Design review of the part built by this model. Coordinates are the model's own, in mm. Give positions to 0.01 mm unless a question says otherwise; leave off trailing zeros. Order: outer loops, then holes, each group sorted by start corner. A loop starts at its lowest first (then second) coordinate and runs counter-clockwise, first axis right, second up. Notation, with made-up numbers: (-10.5, 76.25) - (38.5, 76.25) arc R17 cw to (38.5, 90.25) - close; hole circle Ø6 at (-2.5, 63). An arc over 180 degrees is marked (long way). Write each question's results on one line, items separated by ' | '. Start each with the question number.
```python
from build123d import *

# Parameters (mm, degrees)
SKETCH2_W           = 106
SKETCH2_H           = 106
SKETCH2_R           = 4
SKETCH2_R_2         = 6
BOSS_EXTRUDE1_DEPTH = 25
SKETCH3_W           = 106
SKETCH3_H           = 106
SKETCH3_W_2         = 100
SKETCH3_H_2         = 100
BOSS_EXTRUDE2_DEPTH = 20
SKETCH5_W           = 3
SKETCH5_H           = 23
BOSS_EXTRUDE3_DEPTH = 20
SKETCH7_W           = 20
SKETCH7_H           = 3
BOSS_EXTRUDE4_DEPTH = 20
SKETCH9_R           = 9.905763918
CUT_EXTRUDE1_DEPTH  = 10
SKETCH10_W          = 10
SKETCH10_H          = 4
BOSS_EXTRUDE5_DEPTH = 10
SKETCH11_W          = 10
SKETCH11_H          = 4
BOSS_EXTRUDE6_DEPTH = 10
FILLET2_RADIUS      = 5
FILLET2_LENGTH      = 4
FILLET3_R           = 5
FILLET4_R           = 5
FILLET5_R           = 5
SKETCH13_R          = 1.6
CUT_EXTRUDE2_DEPTH  = 163.397660082
SKETCH14_W          = 35.96051594
SKETCH14_H          = 7.693498276
CUT_EXTRUDE3_DEPTH  = 30


with BuildPart() as part:
    # Sketch2 → Boss-Extrude1 (new body)
    with BuildSketch(Plane(origin=(0, 0, 0), x_dir=(1, 0, 0), z_dir=(0, 1, 0))):
        with Locations((53, 53)):
            Rectangle(SKETCH2_W, SKETCH2_H)
        with Locations(Location((18, 15, 0), (0, 0, 270))):
            Circle(SKETCH2_R, mode=Mode.SUBTRACT)
        with Locations(Location((92, 13.5, 0), (0, 0, 270))):
            Circle(SKETCH2_R_2, mode=Mode.SUBTRACT)
    extrude(amount=BOSS_EXTRUDE1_DEPTH)

    # Sketch3 → Boss-Extrude2 (add)
    with BuildSketch(Plane(origin=(0, 25, 0), x_dir=(1, 0, 0), z_dir=(0, 1, 0))):
        with Locations((53, 53)):
            Rectangle(SKETCH3_W, SKETCH3_H)
        with Locations((53, 53)):
            Rectangle(SKETCH3_W_2, SKETCH3_H_2, mode=Mode.SUBTRACT)
    extrude(amount=BOSS_EXTRUDE2_DEPTH)

    # Sketch5 → Boss-Extrude3 (add)
    with BuildSketch(Plane(origin=(0, 25, 0), x_dir=(1, 0, 0), z_dir=(0, 1, 0))):
        Polygon((3, 28), (3, 25), (36, 25), (36, 23), (39, 23), (39, 43), (36, 43), (36, 28), align=None)
        Polygon((83, 52.5), (83, 26.5), (76, 26.5), (76, 3), (73, 3), (73, 29.5), (80, 29.5), (80, 49.5), (73, 49.5), (73, 52.5), align=None)
        Polygon((3, 63), (3, 60), (29, 60), (29, 80), (26, 80), (26, 63), align=None)
        with Locations((57.5, 14.5)):
            Rectangle(SKETCH5_W, SKETCH5_H)
    extrude(amount=BOSS_EXTRUDE3_DEPTH)

    # Sketch7 → Boss-Extrude4 (add)
    with BuildSketch(Plane(origin=(0, 25, 0), x_dir=(1, 0, 0), z_dir=(0, 1, 0))):
        Polygon((50, 70.496538655), (53, 70.496538655), (53, 73.496538655), (53, 87.496538655), (50, 87.496538655), align=None)
        with Locations((63, 71.996538655)):
            Rectangle(SKETCH7_W, SKETCH7_H)
        Polygon((73, 70.496538655), (73, 52.5), (76, 52.5), (76, 86.5), (73, 86.5), (73, 73.496538655), align=None)
    extrude(amount=BOSS_EXTRUDE4_DEPTH)

    # Sketch9 → Cut-Extrude1 (cut)
    with BuildSketch(Plane(origin=(0, 25, 0), x_dir=(1, 0, 0), z_dir=(0, 1, 0))):
        with Locations(Location((92, 13.5, 0), (0, 0, 270))):
            Circle(SKETCH9_R)
    extrude(amount=-CUT_EXTRUDE1_DEPTH, mode=Mode.SUBTRACT)

    # Sketch10 → Boss-Extrude5 (add)
    with BuildSketch(Plane.XY):
        with Locations((53, 2)):
            Rectangle(SKETCH10_W, SKETCH10_H)
    extrude(amount=BOSS_EXTRUDE5_DEPTH)

    # Sketch11 → Boss-Extrude6 (add)
    with BuildSketch(Plane(origin=(0, 0, -106), x_dir=(-1, 0, 0), z_dir=(0, 0, -1))):
        with Locations((-53, 2)):
            Rectangle(SKETCH11_W, SKETCH11_H)
    extrude(amount=BOSS_EXTRUDE6_DEPTH)

    # Fillet2: full round fillet: the end face becomes a half cylinder, R = half its width
    fillet2_face = Plane((53, 2, -116), x_dir=(0, -1, 0), z_dir=(0, 0, -1))  # on the end face: x along it, z out of the body
    fillet2_slab = fillet2_face.offset(-FILLET2_RADIUS / 2) * Box(FILLET2_LENGTH, 2 * FILLET2_RADIUS, FILLET2_RADIUS, mode=Mode.PRIVATE)  # the body's end, R deep
    fillet2_round = Plane((53, 2, -111), x_dir=(0, 0, -1), z_dir=(0, -1, 0)) * Cylinder(FILLET2_RADIUS, FILLET2_LENGTH, mode=Mode.PRIVATE)  # its axis R under the face
    add(fillet2_slab - fillet2_round, mode=Mode.SUBTRACT)

    # Fillet3
    fillet3_edges = [part.edges().sort_by_distance(p)[0] for p in [
        (48, 2, -106),
        (58, 2, -106),
    ]]
    fillet(fillet3_edges, radius=FILLET3_R - 0.0001)  # a hair under: the kernel refuses the full size

    # Fillet4
    fillet4_edges = [part.edges().sort_by_distance(p)[0] for p in [
        (48, 2, 0),
        (58, 2, 0),
    ]]
    fillet(fillet4_edges, radius=FILLET4_R)

    # Fillet5
    fillet5_edges = [part.edges().sort_by_distance(p)[0] for p in [
        (48, 2, 10),
        (58, 2, 10),
    ]]
    fillet(fillet5_edges, radius=FILLET5_R - 0.0001)  # a hair under: the kernel refuses the full size

    # Sketch13 → Cut-Extrude2 (cut, through all)
    with BuildSketch(Plane(origin=(0, 4, 0), x_dir=(1, 0, 0), z_dir=(0, 1, 0))):
        with Locations(Location((53, -5, 0), (0, 0, 180))):
            Circle(SKETCH13_R)
        with Locations(Location((53, 111, 0), (0, 0, 180))):
            Circle(SKETCH13_R)
    extrude(amount=-CUT_EXTRUDE2_DEPTH, mode=Mode.SUBTRACT)

    # Sketch14 → Cut-Extrude3 (cut)
    with BuildSketch(Plane.XY):
        with Locations((88.01974203, 3.846749138)):
            Rectangle(SKETCH14_W, SKETCH14_H)
    extrude(amount=-CUT_EXTRUDE3_DEPTH, mode=Mode.SUBTRACT)


solid = part.part
```
Q1. Draft analysis for pull direction Z (two halves, no side actions). For faces 1 (the flat face through (3, 35, -14)), 2 (the flat face through (53, 4, 3)), 3 (the cylindrical face through (46, 2, 1)), state which applies: pulls with the +Z half, pulls with the -Z half, needs draft (parallel to the pull), parting line crosses it, or undercut.
Q2. Add section C-C (z = -13.5). Give the number of separate pieces and of enclosed holes in the cut face, plus the area to 3 significant figures.
Q3. Insertion check: pin 1 Ø4 at (x, y) = (56, 34.5) entering from +Z; pin 2 Ø2 at (x, z) = (38, -81.5) entering from +Y; pin 3 Ø8 at (x, z) = (89.5, -60) entering from -Y; pin 4 Ø0.9 at (x, y) = (57.5, 34) entering from -Z. Each pin has a flat end and moves straight along its axis. Give the tip position at first contact, or say it passes through.
Q4. Add section A-A (x = 92). Give the boundary of the cut face in (y, z), plus the area to 3 significant figures.
Q5. Add section B-B (z = -78). Give the boundary of the cut face in (x, y), plus the area to 3 significant figures.
Q6. For line 1 (Z direction, x = 53, y = 1.2); line 2 (X direction, y = 31, z = -44); line 3 (X direction, y = 38, z = -14), list the stretches that pass through material, from the lowest coordinate up. Write a range as [from, to].
Verdict:
1) face 1: undercut | face 2: needs draft | face 3: pulls with the +Z half
2) separate pieces: 3 | enclosed holes: 0 | area: 2,140 mm2
3) pin 1: stops at z = 0 | pin 2: stops at y = 25 | pin 3: stops at y = 0 | pin 4: stops at z = -106
4) outline: (0, -106) - (45, -106) - (45, -103) - (25, -103) - (25, -23.41) - (15, -23.41) - (15, -19.5) - (7.69, -19.5) - (7.69, -30) - (0, -30) - close; (7.69, -7.5) - (15, -7.5) - (15, -3.59) - (25, -3.59) - (25, -3) - (45, -3) - (45, 0) - (7.69, 0) - close | area: 2,250 mm2
5) outline: (0, 0) - (106, 0) - (106, 45) - (103, 45) - (103, 25) - (76, 25) - (76, 45) - (73, 45) - (73, 25) - (53, 25) - (53, 45) - (50, 45) - (50, 25) - (29, 25) - (29, 45) - (26, 45) - (26, 25) - (3, 25) - (3, 45) - (0, 45) - close | area: 2,950 mm2
6) line 1: z = [-116, -112.6], [-109.4, 3.4], [6.6, 10] | line 2: x = [0, 3], [80, 83], [103, 106] | line 3: x = [0, 3], [56, 59], [73, 76], [103, 106]
